Geometry: final body of the model. Coordinates: model frame, mm. Coordinates: 2 decimals unless noted, no trailing zeros. Loops run counter-clockwise (first coordinate to the right, second up) from the corner with the lowest first, then second, coordinate; pieces in that order, holes last. Notation, with made-up numbers: (6.25, 58.25) - (13.25, 58.25) arc R23 ccw to (13.25, 95.25) - close; hole circle Ø11 at (-33, 41). An arc over 180 degrees is marked (long way). Put each result on its own line as item: value. Start each with the question number.
1) Section B-B on y = 25.4. Output: boundary loops of the cut face in (x, z).
2) Section C-C on x = 39. Output: boundary loops of the cut face in (y, z), and give its area (3 significant figures).
3) Contact query for a flat-ended pin moving along its axis: pin 1 Ø6.5 at (x, y) = (209.55, 19.05) entering from +Z. Output: stop coordinate, or through.
4) Section A-A on x = 69.85. Output: boundary loops of the cut face in (y, z).
5) Section D-D on x = 107.95. Output: boundary loops of the cut face in (y, z).
6) Material intervals for line 1 along X through (y, z) = (31.75, 0.85); line 2 along X through (y, z) = (27.5, 0.35); line 3 along X through (y, z) = (30.5, 0.3), sorted ascending. Write a range as from..to.
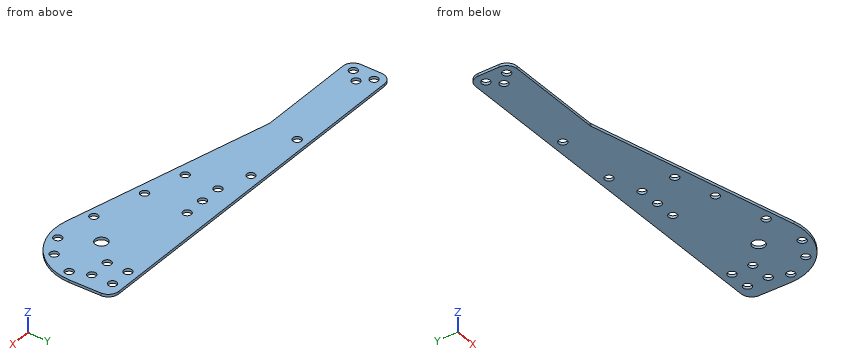
Autodesk Inventor part; units mm, degrees
ref_plane "YZ Plane" through (0, 0, 0) normal (1, 0, 0) x (0, 1, 0)
ref_plane "XZ Plane" through (0, 0, 0) normal (0, 1, 0) x (-1, 0, 0)
ref_plane "XY Plane" through (0, 0, 0) normal (0, 0, 1) x (1, 0, 0)
sketch "Sketch1" plane through (0, 0, 0) normal (0, 0, 1) x (1, 0, 0)
  line L0 (0, 0) -> (247.65, 0)
  line L1 (247.65, 0) -> (247.65, 38.1)
  line L2 (247.65, 38.1) -> (0, 38.1)
  line L3 (0, 38.1) -> (0, 0)
  line L4 (286.1616, 0) -> (255.1962, 0)
  line L5 (255.1962, 0) -> (255.1962, 12.7)
  line L6 (255.1962, 12.7) -> (286.1616, 12.7)
  line L7 (286.1616, 12.7) -> (286.1616, 0)
  line L8 (247.65, 12.7) -> (200.66, 12.7)
  line L9 (16.2468, 38.1) -> (16.2468, 12.7)
  line L10 (16.2468, 12.7) -> (196.85, 12.7)
  line L11 (0, 12.7) -> (17.7951, 12.7)
  circle A0 centre (200.66, 12.7) radius 31.75
  line L12 (232.41, 12.7) -> (231.9451, 38.1)
  line L13 (66.8614, 12.7) -> (200.8653, -20.0324)
  line L14 (193.3963, -18.208) -> (168.91, 12.7)
  point P0 (187.853, -16.3524)
  point P1 (232.3887, 13.8619)
  point P2 (229.7594, 0)
  point P3 (181.61, 38.1)
  point P4 (219.71, 38.1)
  point P5 (171.5606, 0)
  dimension "d0" = 247.65
  dimension "d1" = 38.1
  dimension "d2" = 12.7
  dimension "d3" = 30.9654
  dimension "d4" = 46.99
  dimension "d10" = 25.4
  dimension "d54" = 63.5
extrude "Extrusion4" add sketch "Sketch1" along normal blind 1.5875 contours L13 L0 A0 | L13 L10 A0 L0 | L3 L2 L9 L11 | A0 L14 L0 | L0 L14 A0 | L10 L9 L2 A0 | L14 L0 A0 | L14 A0 L2 L12 L0 | L2 L12 A0
fillet "Fillet6" radius 6.35 3 edges at (0, 38.1, 0.7937) (0, 12.7, 0.7937) (231.9451, 38.1, 0.7937)
sketch "Sketch4" plane through (0, 0, 1.5875) normal (0, 0, 1) x (1, 0, 0)
  arc A0 (6.35, 38.1) -> (0, 31.75) centre (6.35, 31.75) ccw
  line L0 (6.35, 38.1) -> (6.35, 31.75)
  line L1 (6.35, 31.75) -> (0, 31.75)
  circle A1 centre (6.35, 31.75) radius 2.54
  line L2 (6.35, 31.75) -> (6.35, 19.05)
  circle A2 centre (6.35, 19.05) radius 2.54
  line L3 (6.35, 31.75) -> (57.15, 31.75)
  line L4 (57.15, 31.75) -> (107.95, 31.75)
  line L5 (107.95, 31.75) -> (158.75, 31.75)
  line L6 (158.75, 31.75) -> (209.55, 31.75)
  circle A3 centre (107.95, 31.75) radius 2.54
  circle A4 centre (209.55, 31.75) radius 2.54
  line L7 (57.15, 31.75) -> (57.15, 19.05)
  line L8 (57.15, 19.05) -> (107.95, 19.05)
  line L9 (107.95, 19.05) -> (158.75, 19.05)
  line L10 (158.75, 19.05) -> (209.55, 19.05)
  circle A5 centre (209.55, 19.05) radius 2.54
  line L11 (225.7103, 38.1) -> (6.35, 38.1)
  arc A6 (193.3963, -18.208) -> (232.41, 12.7) centre (200.66, 12.7) ccw
  line L12 (209.55, 31.75) -> (196.85, 31.75)
  line L13 (196.85, 31.75) -> (196.85, 19.05)
  circle A7 centre (196.85, 31.75) radius 2.54
  line L14 (196.85, 19.05) -> (196.85, 6.096)
  circle A8 centre (196.85, 6.096) radius 3.81
  line L15 (57.15, 31.75) -> (69.85, 31.75)
  circle A9 centre (69.85, 31.75) radius 2.54
  point P0 (0, 0)
  point P1 (207.01, 31.75)
  dimension "d60" = 6.35
  dimension "d61" = 5.08
  dimension "d62" = 12.7
  dimension "d63" = 5.08
  dimension "d64" = 50.8
  dimension "d65" = 50.8
  dimension "d66" = 50.8
  dimension "d67" = 50.8
  dimension "d70" = 5.08
  dimension "d72" = 5.08
  dimension "d76" = 5.08
  dimension "d86" = 12.7
  dimension "d88" = 5.08
  dimension "d89" = 12.954
  dimension "d90" = 7.62
  dimension "d116" = 12.7
  dimension "d117" = 5.08
extrude "Extrusion5" cut sketch "Sketch4" against normal blind 25.4 contours A4 | A5 | A8 | A2 | A1 L3 L0 | L0 L1 A1 | L1 L2 A1 | L3 A1 L2 | A9 L4 | L4 A9 | A3 L5 L4 | L4 L5 A3
sketch "Sketch5" plane through (0, 0, 1.5875) normal (0, 0, 1) x (1, 0, 0)
  circle A0 centre (209.55, 31.75) radius 2.54
  line L0 (209.55, 31.75) -> (222.25, 31.75)
  line L1 (222.25, 31.75) -> (222.25, 19.05)
  line L2 (222.25, 19.05) -> (226.6625, 8.5061)
  line L3 (226.6625, 8.5061) -> (219.2036, -6.223)
  line L4 (219.2036, -6.223) -> (207.01, -13.0403)
  line L5 (207.01, -13.0403) -> (181.8398, -9.6316)
  line L6 (181.8398, -9.6316) -> (151.2071, -1.2828)
  line L7 (151.2071, -1.2828) -> (126.701, 5.3962)
  circle A1 centre (126.701, 5.3962) radius 2.54
  circle A2 centre (151.2071, -1.2828) radius 2.54
  circle A3 centre (181.8398, -9.6316) radius 2.54
  circle A4 centre (207.01, -13.0403) radius 2.54
  circle A5 centre (219.2036, -6.223) radius 2.54
  circle A6 centre (226.6625, 8.5061) radius 2.54
  circle A7 centre (222.25, 19.05) radius 2.54
  circle A8 centre (222.25, 31.75) radius 2.54
  circle A9 centre (6.35, 19.05) radius 2.54
  line L8 (6.35, 19.05) -> (15.3303, 28.0303)
  line L9 (6.35, 19.05) -> (19.05, 19.05) construction
  circle A10 centre (6.35, 31.75) radius 2.54
  line L10 (6.35, 31.75) -> (15.3303, 22.7697)
  line L11 (6.35, 31.75) -> (19.05, 31.75) construction
  circle A11 centre (12.7, 25.4) radius 2.54
  line L12 (126.701, 5.3962) -> (126.701, 25.4)
  line L13 (126.701, 25.4) -> (139.401, 25.4)
  line L14 (139.401, 25.4) -> (152.101, 25.4)
  circle A12 centre (126.701, 25.4) radius 2.54
  circle A13 centre (139.401, 25.4) radius 2.54
  circle A14 centre (152.101, 25.4) radius 2.54
  point P0 (0, 0)
  dimension "d91" = 12.7
  dimension "d92" = 12.7
  dimension "d93" = 11.43
  dimension "d94" = 16.51
  dimension "d95" = 13.97
  dimension "d96" = 25.4
  dimension "d97" = 31.75
  dimension "d98" = 25.4
  dimension "d99" = 5.08
  dimension "d100" = 5.08
  dimension "d101" = 5.08
  dimension "d102" = 5.08
  dimension "d103" = 5.08
  dimension "d104" = 5.08
  dimension "d105" = 5.08
  dimension "d106" = 5.08
  dimension "d109" = 12.7
  dimension "d110" = 45
  dimension "d111" = 12.7
  dimension "d112" = 45
  dimension "d113" = 5.08
  dimension "d129" = 12.7
  dimension "d130" = 12.7
  dimension "d131" = 5.08
  dimension "d132" = 5.08
  dimension "d133" = 5.08
extrude "Extrusion6" cut sketch "Sketch5" against normal blind 25.4 contours A14 | A13 L14 L13 | L13 L14 A13 | A12 L13 L12 | L12 L13 A12 | A1 L12 L7 | L7 L12 A1 | A2 L7 L6 | L6 L7 A2 | A3 L6 L5 | L5 L6 A3 | A4 L5 L4 | L4 L5 A4 | A5 L4 L3 | L3 L4 A5 | A6 L3 L2 | L2 L3 A6 | A7 L2 L1 | L1 L2 A7 | A8 L1 L0 | L0 L1 A8 | A11 L10 L8 | L8 L10 A11 | L10 A11 L8 | L8 A11 L10
fillet "Fillet7" radius 3.175 1 edges at (66.8614, 12.7, 0.7937)
properties part number "intake sled v5"
Answer block:
1. outline: (0, 0) - (10.16, 0) - (10.16, 1.59) - (0, 1.59) - close; (15.24, 0) - (124.16, 0) - (124.16, 1.59) - (15.24, 1.59) - close; (129.24, 0) - (136.86, 0) - (136.86, 1.59) - (129.24, 1.59) - close; (141.94, 0) - (149.56, 0) - (149.56, 1.59) - (141.94, 1.59) - close; (154.64, 0) - (232.18, 0) - (232.18, 1.59) - (154.64, 1.59) - close
2. outline: (12.7, 0) - (38.1, 0) - (38.1, 1.59) - (12.7, 1.59) - close
2. area: 40.3 mm²
3. pin 1: stops at z = 1.59
4. outline: (11.97, 0) - (29.21, 0) - (29.21, 1.59) - (11.97, 1.59) - close; (34.29, 0) - (38.1, 0) - (38.1, 1.59) - (34.29, 1.59) - close
5. outline: (2.66, 0) - (29.21, 0) - (29.21, 1.59) - (2.66, 1.59) - close; (34.29, 0) - (38.1, 0) - (38.1, 1.59) - (34.29, 1.59) - close
6. line 1: x = 0..3.81, 8.89..67.31, 72.39..105.41, 110.49..207.01, 212.09..219.71, 224.79..232.06
6. line 2: x = 0..11.27, 14.13..125.27, 128.13..137.97, 140.83..150.67, 153.53..232.14
6. line 3: x = 0..4.14, 8.56..67.64, 72.06..105.74, 110.16..207.34, 211.76..220.04, 224.46..232.08
